from build123d import *

# Parameters (mm, degrees)
SZKIC1_W                    = 460
SZKIC1_H                    = 580
SZKIC1_W_2                  = 400
SZKIC1_H_2                  = 520
DODANIE_WYCI_GNI_CIE1_DEPTH = 30
SZKIC4_R                    = 2.5
WYTNIJ_WYCI_GNI_CIE2_DEPTH  = 5
SZKIC5_W                    = 30
SZKIC5_H                    = 30
DODANIE_WYCI_GNI_CIE3_DEPTH = 330
DODANIE_WYCI_GNI_CIE4_REACH = 698.419
SZKIC6_W                    = 30
SZKIC6_H                    = 30
DODANIE_WYCI_GNI_CIE5_REACH = 698.419
SZKIC7_W                    = 30
SZKIC7_H                    = 30
SZKIC8_W                    = 30
SZKIC8_H                    = 30
DODANIE_WYCI_GNI_CIE6_DEPTH = 330
DODANIE_WYCI_GNI_CIE7_REACH = 633.348
SZKIC9_W                    = 30
SZKIC9_H                    = 30
DODANIE_WYCI_GNI_CIE8_REACH = 698.419
SZKIC10_W                   = 30
SZKIC10_H                   = 30
SZKIC11_R                   = 2
WYTNIJ_WYCI_GNI_CIE3_DEPTH  = 5
SZKIC12_R                   = 2
WYTNIJ_WYCI_GNI_CIE4_DEPTH  = 5
SZKIC2_R                    = 2
WYTNIJ_WYCI_GNI_CIE5_DEPTH  = 5
LUSTRO2_COPY_1_SKETCH_R     = 2
LUSTRO2_COPY_1_DEPTH        = 5


with BuildPart() as part:
    # Szkic1 → Dodanie-wyciągnięcie1 (new body)
    with BuildSketch(Plane.XY):
        Rectangle(SZKIC1_W, SZKIC1_H)
        Rectangle(SZKIC1_W_2, SZKIC1_H_2, mode=Mode.SUBTRACT)
    extrude(amount=DODANIE_WYCI_GNI_CIE1_DEPTH)

    # Szkic4 → Wytnij-wyciągnięcie2 (cut)
    with BuildSketch(Plane.XY.offset(30)):
        with Locations((215, 45)):
            Circle(SZKIC4_R)
        with Locations((215, -45)):
            Circle(SZKIC4_R)
    extrude(amount=-WYTNIJ_WYCI_GNI_CIE2_DEPTH, mode=Mode.SUBTRACT)

    # Szkic5 → Dodanie-wyciągnięcie3 (add)
    with BuildSketch(Plane.XY.offset(30)):
        with Locations((30, -275)):
            Rectangle(SZKIC5_W, SZKIC5_H)
        with Locations((30, 275)):
            Rectangle(SZKIC5_W, SZKIC5_H)
    extrude(amount=DODANIE_WYCI_GNI_CIE3_DEPTH)

    # Szkic6 → Dodanie-wyciągnięcie4 (add, up to next)
    with BuildSketch(Plane.XZ.offset(-260), mode=Mode.PRIVATE) as dodanie_wyci_gni_cie4_sk1:
        with Locations((30, 245)):
            Rectangle(SZKIC6_W, SZKIC6_H)
    dodanie_wyci_gni_cie4_tool1 = extrude(dodanie_wyci_gni_cie4_sk1.sketch, amount=DODANIE_WYCI_GNI_CIE4_REACH, mode=Mode.PRIVATE) - part.part
    add(dodanie_wyci_gni_cie4_tool1.solids().sort_by_distance((30, 260, 245))[0])

    # Szkic7 → Dodanie-wyciągnięcie5 (add, up to next)
    with BuildSketch(Plane(origin=(0, 260, 0), x_dir=(-1, 0, 0), z_dir=(0, -1, 0)), mode=Mode.PRIVATE) as dodanie_wyci_gni_cie5_sk1:
        with Locations((-30, -345)):
            Rectangle(SZKIC7_W, SZKIC7_H)
    dodanie_wyci_gni_cie5_tool1 = extrude(dodanie_wyci_gni_cie5_sk1.sketch, amount=DODANIE_WYCI_GNI_CIE5_REACH, mode=Mode.PRIVATE) - part.part
    add(dodanie_wyci_gni_cie5_tool1.solids().sort_by_distance((30, 260, 345))[0])

    # Szkic8 → Dodanie-wyciągnięcie6 (add)
    with BuildSketch(Plane.XY.offset(30)):
        with Locations((-215, 275)):
            Rectangle(SZKIC8_W, SZKIC8_H)
        with Locations((-215, -275)):
            Rectangle(SZKIC8_W, SZKIC8_H)
    extrude(amount=DODANIE_WYCI_GNI_CIE6_DEPTH)

    # Szkic9 → Dodanie-wyciągnięcie7 (add, up to next)
    with BuildSketch(Plane(origin=(-200, 0, 0), x_dir=(0, 0, -1), z_dir=(1, 0, 0)), mode=Mode.PRIVATE) as dodanie_wyci_gni_cie7_sk1:
        with Locations((-345, 275)):
            Rectangle(SZKIC9_W, SZKIC9_H)
    dodanie_wyci_gni_cie7_tool1 = extrude(dodanie_wyci_gni_cie7_sk1.sketch, amount=DODANIE_WYCI_GNI_CIE7_REACH, mode=Mode.PRIVATE) - part.part
    # Szkic9 → Dodanie-wyciągnięcie7 (add, up to next)
    with BuildSketch(Plane(origin=(-200, 0, 0), x_dir=(0, 0, -1), z_dir=(1, 0, 0)), mode=Mode.PRIVATE) as dodanie_wyci_gni_cie7_sk2:
        with Locations((-345, -275)):
            Rectangle(SZKIC9_W, SZKIC9_H)
    dodanie_wyci_gni_cie7_tool2 = extrude(dodanie_wyci_gni_cie7_sk2.sketch, amount=DODANIE_WYCI_GNI_CIE7_REACH, mode=Mode.PRIVATE) - part.part
    add(dodanie_wyci_gni_cie7_tool1.solids().sort_by_distance((-200, 275, 345))[0])
    add(dodanie_wyci_gni_cie7_tool2.solids().sort_by_distance((-200, -275, 345))[0])

    # Szkic10 → Dodanie-wyciągnięcie8 (add, up to next)
    with BuildSketch(Plane.XZ.offset(-260), mode=Mode.PRIVATE) as dodanie_wyci_gni_cie8_sk1:
        with Locations((-215, 345)):
            Rectangle(SZKIC10_W, SZKIC10_H)
    dodanie_wyci_gni_cie8_tool1 = extrude(dodanie_wyci_gni_cie8_sk1.sketch, amount=DODANIE_WYCI_GNI_CIE8_REACH, mode=Mode.PRIVATE) - part.part
    add(dodanie_wyci_gni_cie8_tool1.solids().sort_by_distance((-215, 260, 345))[0])

    # Szkic11 → Wytnij-wyciągnięcie3 (cut)
    with BuildSketch(Plane.ZY.offset(-15)):
        with Locations((245, 25)):
            Circle(SZKIC11_R)
        with Locations((245, -25)):
            Circle(SZKIC11_R)
    extrude(amount=-WYTNIJ_WYCI_GNI_CIE3_DEPTH, mode=Mode.SUBTRACT)

    # Szkic12 → Wytnij-wyciągnięcie4 (cut)
    with BuildSketch(Plane.XY.offset(360)):
        with Locations((30, -45)):
            Circle(SZKIC12_R)
        with Locations((30, 45)):
            Circle(SZKIC12_R)
    extrude(amount=-WYTNIJ_WYCI_GNI_CIE4_DEPTH, mode=Mode.SUBTRACT)

    # Szkic2 → Wytnij-wyciągnięcie5 (cut)
    with BuildSketch(Plane.XY.offset(30)):
        with Locations((215, 198)):
            Circle(SZKIC2_R)
        with Locations((215, 158)):
            Circle(SZKIC2_R)
    wytnij_wyci_gni_cie5 = extrude(amount=-WYTNIJ_WYCI_GNI_CIE5_DEPTH, mode=Mode.SUBTRACT)

    # Lustro1: Wytnij-wyciągnięcie5 across plane
    add(wytnij_wyci_gni_cie5.mirror(Plane(origin=(0, 0, 0), x_dir=(0, 0, 1), z_dir=(1, 0, 0))), mode=Mode.SUBTRACT)

    # Lustro2: Wytnij-wyciągnięcie5 across plane
    add(wytnij_wyci_gni_cie5.mirror(Plane.ZX), mode=Mode.SUBTRACT)

    # Lustro2 copy 1 sketch → Lustro2 copy 1 (cut)
    with BuildSketch(Plane(origin=(0, 0, 30), x_dir=(-1, 0, 0), z_dir=(0, 0, 1))):
        with Locations((215, 198)):
            Circle(LUSTRO2_COPY_1_SKETCH_R)
        with Locations((215, 158)):
            Circle(LUSTRO2_COPY_1_SKETCH_R)
    extrude(amount=-LUSTRO2_COPY_1_DEPTH, mode=Mode.SUBTRACT)


solid = part.part
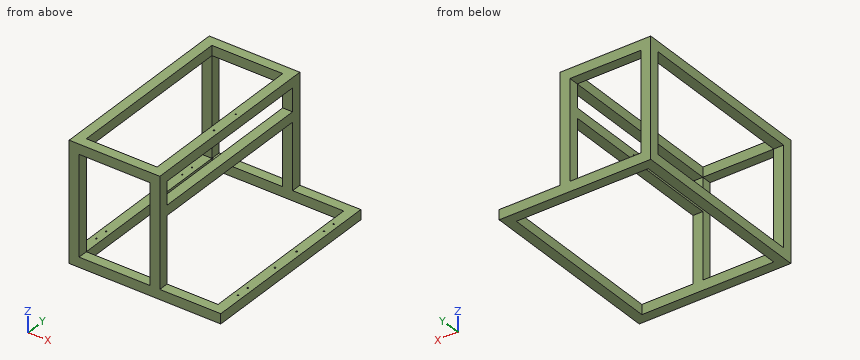
Design review of the part built by this model. Coordinates are the model's own, in mm. Give positions to 0.01 mm unless a question says otherwise; leave off trailing zeros. Loops run counter-clockwise (first coordinate to the right, second up) from the corner with the lowest first, then second, coordinate; pieces in that order, holes last. Notation, with made-up numbers: (57, 29) - (81, 29) arc R34 ccw to (81, 67) - close; hole circle Ø4 at (76.5, 64). An arc over 180 degrees is marked (long way). Write item = value, one per line.
1) Take a section at B-B on z = 276. State the section outline as (x, y) points.
Result sheet:
outline = (-230, -290) - (-200, -290) - (-200, -260) - (-230, -260) - close; (-230, 260) - (-200, 260) - (-200, 290) - (-230, 290) - close; (15, -290) - (45, -290) - (45, -260) - (15, -260) - close; (15, 260) - (45, 260) - (45, 290) - (15, 290) - close
2) Clearance check with flat-ended pins moving along their axes: pin 1 Ø3.5 at (y, z) = (25, 245) entering from -X; pin 2 Ø15 at (x, y) = (36, -119.5) entering from -Z; pin 3 Ø6 at (x, y) = (215, 45) entering from +Z. State where each tip first meets the part, or that it passes through.
Result sheet:
pin_1 = 20
pin_2 = 230
pin_3 = 30
3) To check wall thickness, follow line 1 (Y direction, x = 18.1, z = 245); line 2 (Y direction, x = -215, z = 27); line 3 (Z direction, x = 24.5, y = -69.5). State the ranges of each line that lie inside material, in increasing order.
Result sheet:
line_1 = -290 to -27, -23 to 23, 27 to 290
line_2 = -290 to -200, -196 to -160, -156 to 156, 160 to 196, 200 to 290
line_3 = 230 to 260, 330 to 360
4) Take a section at D-D on x = -24.5. State the section outline as (y, z) points, and give its area (3 significant figures).
Result sheet:
outline = (-290, 0) - (-260, 0) - (-260, 30) - (-290, 30) - close; (-290, 330) - (-260, 330) - (-260, 360) - (-290, 360) - close; (260, 0) - (290, 0) - (290, 30) - (260, 30) - close; (260, 330) - (290, 330) - (290, 360) - (260, 360) - close
area = 3,600 mm2
5) Take a section at C-C on y = 188. State the section outline as (x, z) points, and give its area (3 significant figures).
Result sheet:
outline = (-230, 0) - (-200, 0) - (-200, 30) - (-230, 30) - close; (-230, 330) - (-200, 330) - (-200, 360) - (-230, 360) - close; (15, 230) - (45, 230) - (45, 260) - (15, 260) - close; (15, 330) - (45, 330) - (45, 360) - (15, 360) - close; (200, 0) - (230, 0) - (230, 30) - (200, 30) - close
area = 4,500 mm2
6) Take a section at A-A on x = 125. State the section outline as (y, z) points, and give its area (3 significant figures).
Result sheet:
outline = (-290, 0) - (-260, 0) - (-260, 30) - (-290, 30) - close; (260, 0) - (290, 0) - (290, 30) - (260, 30) - close
area = 1,800 mm2
